Source: CAD feature listing. Evaluate the final solid. Frame: model axes, mm. Coordinates: 2 decimals unless noted, no trailing zeros. Loops run counter-clockwise (first coordinate to the right, second up) from the corner with the lowest first, then second, coordinate; pieces in that order, holes last.
Item 1: Section query C-C, the plane x = -61. Return the cut outline in (y, z).
Item 2: Pin query (flat end, axial travel): pin 1 Ø3 at (x, z) = (-8.5, -9.5) entering from +Y. Return the tip coordinate at first contact, or that it passes through.
Item 3: Pull-direction query (X, two-part tool) for faces 1 (the cylindrical face through (67.648, -0.74, 32.566)), 2 (the cylindrical face through (67.648, -0.74, -33.434)), 3 (the flat face through (-1, -1.5, -1)); classes: +X half, -X half, draft (parallel to the pull), parting line (faces both ways), or undercut.
Item 4: Section query D-D, the plane x = 69.6. Return the cut outline in (y, z), then the cut area to 3 significant figures.
Item 5: Line query: probe 1 along X at (y, z) = (-0.5, 33); probe 2 along X at (y, z) = (-1.05, 26.5); probe 3 along Z at (x, y) = (-37, -0.75). Output: solid intervals per line, ascending.
Item 6: Section query A-A, the plane z = 23.5. Return the cut outline in (x, y).
Item 7: Section query B-B, the plane y = -0.95. Return the cut outline in (x, z), then the cut area to 3 significant figures.
```python
from build123d import *

# Parameters (mm, degrees)
SKETCH1_W           = 149.2
SKETCH1_H           = 76
SKETCH1_R           = 2
SKETCH1_W_2         = 49.8
SKETCH1_H_2         = 8.25
BOSS_EXTRUDE1_DEPTH = 1.5


with BuildPart() as part:
    # Sketch1 → Boss-Extrude1 (new body)
    with BuildSketch(Plane(origin=(0, 0, 0), x_dir=(1, 0, 0), z_dir=(0, 1, 0))):
        Rectangle(SKETCH1_W, SKETCH1_H)
        with Locations(Location((-69.6, 33, 0), (0, 0, 270))):
            Circle(SKETCH1_R, mode=Mode.SUBTRACT)
        with Locations(Location((69.6, 33, 0), (0, 0, 270))):
            Circle(SKETCH1_R, mode=Mode.SUBTRACT)
        with Locations(Location((69.6, -33, 0), (0, 0, 270))):
            Circle(SKETCH1_R, mode=Mode.SUBTRACT)
        with Locations(Location((-69.6, -33, 0), (0, 0, 270))):
            Circle(SKETCH1_R, mode=Mode.SUBTRACT)
        with Locations((-41.7, -24.875)):
            Rectangle(SKETCH1_W_2, SKETCH1_H_2, mode=Mode.SUBTRACT)
        with Locations((15.35, -24.875)):
            Rectangle(SKETCH1_W_2, SKETCH1_H_2, mode=Mode.SUBTRACT)
    extrude(amount=-BOSS_EXTRUDE1_DEPTH)


solid = part.part
```
Verdict:
1. outline: (-1.5, -38) - (0, -38) - (0, 20.75) - (-1.5, 20.75) - close; (-1.5, 29) - (0, 29) - (0, 38) - (-1.5, 38) - close
2. pin 1: stops at y = 0
3. face 1: undercut
3. face 2: undercut
3. face 3: draft
4. outline: (-1.5, -38) - (0, -38) - (0, -35) - (-1.5, -35) - close; (-1.5, -31) - (0, -31) - (0, 31) - (-1.5, 31) - close; (-1.5, 35) - (0, 35) - (0, 38) - (-1.5, 38) - close
4. area: 102 mm2
5. probe 1: x = -74.6 to -71.6, -67.6 to 67.6, 71.6 to 74.6
5. probe 2: x = -74.6 to -66.6, -16.8 to -9.55, 40.25 to 74.6
5. probe 3: z = -38 to 20.75, 29 to 38
6. outline: (-74.6, -1.5) - (-66.6, -1.5) - (-66.6, 0) - (-74.6, 0) - close; (-16.8, -1.5) - (-9.55, -1.5) - (-9.55, 0) - (-16.8, 0) - close; (40.25, -1.5) - (74.6, -1.5) - (74.6, 0) - (40.25, 0) - close
7. outline: (-74.6, -38) - (74.6, -38) - (74.6, 38) - (-74.6, 38) - close; hole circle Ø4 at (-69.6, -33); hole circle Ø4 at (-69.6, 33); hole (-66.6, 20.75) - (-16.8, 20.75) - (-16.8, 29) - (-66.6, 29) - close; hole (-9.55, 20.75) - (40.25, 20.75) - (40.25, 29) - (-9.55, 29) - close; hole circle Ø4 at (69.6, -33); hole circle Ø4 at (69.6, 33)
7. area: 10,500 mm2
